```python
from build123d import *

# Parameters (mm, degrees)
F0_W      = 64.6
F0_H      = 37.6
F1_DEPTH  = 28
F3_DEPTH  = 1.5
F4_W      = 1.5
F4_H      = 1.5
F5_DEPTH  = 22
F6_T      = -1.5
F7_W      = 64.6
F7_H      = 2.5
F8_DEPTH  = 1.5
F9_W      = 5
F9_H      = 2
F10_DEPTH = 31.6
F11_W     = 3.2
F11_H     = 3.8
F12_DEPTH = 1.5
F14_DEPTH = 38.901
F15_W     = 16
F15_H     = 11.4
F15_W_2   = 11
F16_DEPTH = 9.4
F17_R     = 1
F18_R     = 0.5


# Not quite as in the source:
# - two fillets or chamfers of one size are made in one step
# - a pattern or mirror of a feature is missing from the dataset's text; its kind, count and spacing are read off the source's solid


with BuildPart() as f1:
    # F0 (on Top) → F1 (new body)
    with BuildSketch(Plane.XY):
        Rectangle(F0_W, F0_H)
    extrude(amount=F1_DEPTH)

    # F2 (on face) → F3 (cut)
    with BuildSketch(Plane.XZ.offset(18.8)):
        Polygon((-13.0391832353, 0), (-8.6608167647, 0), (-9.25, 22.5), (-12.45, 22.5), align=None)
        Polygon((12.45, 22.5), (9.25, 22.5), (8.6608167647, 0), (13.0391832353, 0), align=None)
    f3 = extrude(amount=-F3_DEPTH, mode=Mode.SUBTRACT)

    # F3_copies: F3 across plane
    add(f3.mirror(Plane.ZX), mode=Mode.SUBTRACT)

    # F4 (on face) → F5 (cut)
    with BuildSketch(Plane(origin=(0, 0, 0), x_dir=(1, 0, 0), z_dir=(0, 0, -1))):
        with Locations((-31.55, 18.05)):
            Rectangle(F4_W, F4_H)
        with Locations((31.55, 18.05)):
            Rectangle(F4_W, F4_H)
        with Locations((31.55, -18.05)):
            Rectangle(F4_W, F4_H)
        with Locations((-31.55, -18.05)):
            Rectangle(F4_W, F4_H)
    extrude(amount=-F5_DEPTH, mode=Mode.SUBTRACT)

    # F6
    f6_openings = [f1.faces().sort_by_distance(p)[0] for p in [
        (0, 0, 28),
    ]]
    offset(amount=F6_T, openings=f6_openings, kind=Kind.INTERSECTION)

    # F7 (on face) → F8 (join)
    with BuildSketch(Plane.XY.offset(28)):
        with Locations((0, -20.05)):
            Rectangle(F7_W, F7_H)
        with Locations((0, 20.05)):
            Rectangle(F7_W, F7_H)
    extrude(amount=-F8_DEPTH)

    # F9 (on Right) → F10 (cut, symmetric)
    with BuildSketch(Plane.YZ):
        with Locations((-14.8, 26.2)):
            Rectangle(F9_W, F9_H)
        with Locations((14.8, 26.2)):
            Rectangle(F9_W, F9_H)
    extrude(amount=F10_DEPTH, both=True, mode=Mode.SUBTRACT)

    # F11 (on face) → F12 (join)
    with BuildSketch(Plane.XZ.offset(18.8)):
        with Locations((-5, 21.1)):
            Rectangle(F11_W, F11_H)
        with Locations((5, 21.1)):
            Rectangle(F11_W, F11_H)
    f12 = extrude(amount=F12_DEPTH)

    # F12_copies: F12 across plane
    add(f12.mirror(Plane.ZX))

    # F13 (on face) → F14 (cut, through all)
    with BuildSketch(Plane.YZ.offset(6.6)):
        Polygon((-18.8, 19.2), (-20.3, 23), (-20.3, 19.2), align=None)
    f14 = extrude(amount=-F14_DEPTH, mode=Mode.SUBTRACT)

    # F14_copies: F14 across plane
    add(f14.mirror(Plane.ZX), mode=Mode.SUBTRACT)

    # F15 (on face) → F16 (cut)
    with BuildSketch(Plane(origin=(0, 0, 0), x_dir=(1, 0, 0), z_dir=(0, 0, -1))):
        with Locations((0, 13.1)):
            Rectangle(F15_W, F15_H)
        with Locations((21.7, 13.1)):
            Rectangle(F15_W_2, F15_H)
    extrude(amount=-F16_DEPTH, mode=Mode.SUBTRACT)

    # F17
    f17_edges = [f1.edges().sort_by_distance(p)[0] for p in [
        (32.3, -21.3, 27.25),
        (32.3, 21.3, 27.25),
        (-32.3, -21.3, 27.25),
        (-32.3, 21.3, 27.25),
    ]]
    fillet(f17_edges, radius=F17_R)

    # F18
    f18_edges = [f1.edges().sort_by_distance(p)[0] for p in [
        (32.3, 0, 0),
        (29, -18.8, 0),
        (14.619592, -18.8, 0),
        (-8.330408, -18.8, 0),
        (-21.919592, -18.8, 0),
        (-32.3, 0, 0),
        (0, 18.8, 0),
        (8.330408, -18.8, 0),
        (-21.919592, 18.8, 0),
        (21.919592, 18.8, 0),
        (30.8, 0, 1.5),
        (-21.900209, -17.3, 1.5),
        (28.25, -17.3, 1.5),
        (-30.8, 0, 1.5),
        (-21.900209, 17.3, 1.5),
        (0, 17.3, 1.5),
        (21.900209, 17.3, 1.5),
        (29.3, -16.55, 1.5),
        (14.500419, -16.55, 1.5),
        (11.250209, -15.8, 1.5),
        (-11.250209, -15.8, 1.5),
        (-14.500419, -16.55, 1.5),
        (-29.3, -16.55, 1.5),
        (-30.05, -15.8, 1.5),
        (-30.05, 15.8, 1.5),
        (-29.3, 16.55, 1.5),
        (-14.500419, 16.55, 1.5),
        (-10.85, 15.8, 1.5),
        (-7.199581, 16.55, 1.5),
        (7.199581, 16.55, 1.5),
        (10.85, 15.8, 1.5),
        (14.500419, 16.55, 1.5),
        (29.3, 16.55, 1.5),
        (30.05, 15.8, 1.5),
        (30.05, -15.8, 1.5),
    ]]
    fillet(f18_edges, radius=F18_R)


solid = f1.part
```
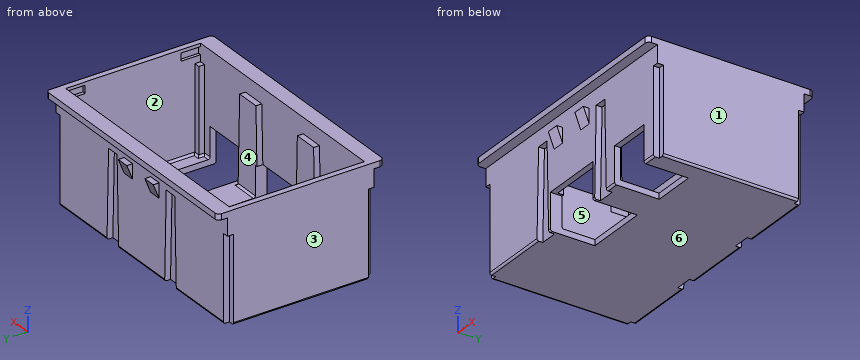
Could you check a few things on this model? Use its own coordinates, in mm. Face numbers are marked on the shaded views. A direction names the side the tool comes from. Coordinates: 2 decimals unless noted, no trailing zeros. Write each loop counter-clockwise with the first axis right and the second up, starting at its lowest first coordinate (ties: lowest second). Pieces come first, ordered by that corner, then holes. Notation, with made-up numbers: (-23, 1.25) -> (18, 1.25) arc R20 cw to (18, 23.25) -> close; hole circle Ø6 at (40.5, -4.75). An arc over 180 degrees is marked (long way). Return JSON: item names as keys, results as strings.
(1) I'm going to push flat-ended pins straight in: pin 1 (3 mm diameter, centred on x = -21.5, z = 4, fed in from +Y); pin 2 (1 mm diameter, centred on x = 11.5, y = 7.5, fed in from -Z); pin 3 (2 mm diameter, centred on x = 10.5, z = 12, fed in from +Y); pin 4 (4 mm diameter, centred on x = -8, y = 9.5, fed in from +Z). Where does each tip first touch, or does it pass through?
Numbers:
{"pin 1": "stops at y = 18.8", "pin 2": "stops at z = 0", "pin 3": "stops at y = 17.3", "pin 4": "stops at z = 1.5"}
(2) Imagine slicing it at A-A, the plane x = -1. Please give me the cut outline in (y, z), then the cut area to 3 significant figures.
Numbers:
{"outline": "(-21.3, 26.5) -> (-18.8, 26.5) -> (-18.8, 9.4) -> (-17.3, 9.4) -> (-17.3, 28) -> (-21.3, 28) -> close; (-7.4, 0) -> (18.3, 0) arc R0.5 ccw to (18.8, 0.5) -> (18.8, 26.5) -> (21.3, 26.5) -> (21.3, 28) -> (17.3, 28) -> (17.3, 2) arc R0.5 cw to (16.8, 1.5) -> (-7.4, 1.5) -> close", "area": "114 mm2"}
(3) Which directions (+Z, -Z, +X, -X, +Y, -Y) give clear straight access to the entire face, cutting with the end or side of a thin tool? Please do the marked faces 1 and 2.
Numbers:
{"face 1": "+Z, -Z, +X, +Y, -Y", "face 2": "+Z"}
(4) I need wall thicknesses on L1, parallel to Y at x = -17.5, z = 25.5; L2, parallel to X at y = -15, z = 12; L3, parallel to X at y = -18.5, z = 11.75. Which ranges of each line are inside material? Lowest first, please.
Numbers:
{"L1": "y = -18.8 to -17.3, 17.3 to 18.8", "L2": "x = -32.3 to -30.8, 30.8 to 32.3", "L3": "x = -30.8 to -12.73, -8.97 to 8.97, 12.73 to 30.8"}
(5) We'd pull the mould along X, two halves only. Please class the marked faces 3, 4, 5 and 6: +X half, -X half, draft (parallel to the pull), parting line (faces both ways), or undercut.
Numbers:
{"face 3": "-X half", "face 4": "undercut", "face 5": "undercut", "face 6": "draft"}
(6) Imagine slicing it at C-C, the plane x = -17.5. Please give me the cut outline in (y, z).
Numbers:
{"outline": "(-21.3, 26.5) -> (-18.8, 26.5) -> (-18.8, 0.5) arc R0.5 ccw to (-18.3, 0) -> (18.3, 0) arc R0.5 ccw to (18.8, 0.5) -> (18.8, 26.5) -> (21.3, 26.5) -> (21.3, 28) -> (17.3, 28) -> (17.3, 2) arc R0.5 cw to (16.8, 1.5) -> (-16.8, 1.5) arc R0.5 cw to (-17.3, 2) -> (-17.3, 28) -> (-21.3, 28) -> close"}
(7) Imagine slicing it at B-B, the plane y = -10. Please give me the cut outline in (x, z).
Numbers:
{"outline": "(-32.3, 0.5) arc R0.5 ccw to (-31.8, 0) -> (-8, 0) -> (-8, 1.5) -> (-30.3, 1.5) arc R0.5 cw to (-30.8, 2) -> (-30.8, 28) -> (-32.3, 28) -> close; (8, 0) -> (16.2, 0) -> (16.2, 1.5) -> (8, 1.5) -> close; (27.2, 0) -> (31.8, 0) arc R0.5 ccw to (32.3, 0.5) -> (32.3, 28) -> (30.8, 28) -> (30.8, 2) arc R0.5 cw to (30.3, 1.5) -> (27.2, 1.5) -> close"}
